```python
from build123d import *

# Parameters (mm, degrees)
BASE_W                = 83
BASE_H                = 80
MAIN_DEPTH            = 5
GEAR_AXIS_HOLES_D     = 5.8
CHAMFER1_SIZE         = 15
FILLET6_R             = 3
F_4_CLEARANCE_HOLE1_D = 3.2639


with BuildPart() as part:
    # Base → Main (new body)
    with BuildSketch(Plane.XY):
        with Locations((1.724154817, 0)):
            Rectangle(BASE_W, BASE_H)
    extrude(amount=MAIN_DEPTH)

    # Gear Axis Holes (through all)
    with Locations(Plane(origin=(0, 0, 5), x_dir=(-1, 0, 0), z_dir=(0, 0, 1))):
        with Locations((22.275845183, 20), (22.275845183, -20)):
            Hole(GEAR_AXIS_HOLES_D / 2)

    # Chamfer1
    chamfer1_edges = [part.edges().sort_by_distance(p)[0] for p in [
        (-39.775845183, -40, 2.5),
        (-39.775845183, 40, 2.5),
    ]]
    chamfer(chamfer1_edges, length=CHAMFER1_SIZE)

    # Fillet6
    fillet6_edges = [part.edges().sort_by_distance(p)[0] for p in [
        (-24.775845183, -40, 2.5),
        (-39.775845183, 25, 2.5),
        (-39.775845183, -25, 2.5),
        (-24.775845183, 40, 2.5),
        (43.224154817, 40, 2.5),
        (43.224154817, -40, 2.5),
    ]]
    fillet(fillet6_edges, radius=FILLET6_R)

    # #4 Clearance Hole1 (through all)
    with Locations(Plane.XY.offset(5)):
        with Locations((13.224154817, 35), (38.224154817, 35), (38.224154817, -35)):
            Hole(F_4_CLEARANCE_HOLE1_D / 2)


solid = part.part
```
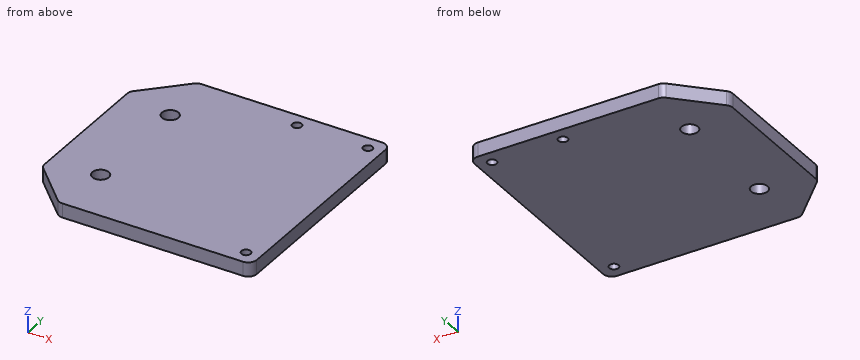
Design review of the part built by this model. Coordinates are the model's own, in mm. Round coordinates to 2 decimals unless told otherwise and drop trailing zeros. Write each loop counter-clockwise with the first axis right and the second up, starting at its lowest first coordinate (ties: lowest second). Pieces come first, ordered by that corner, then holes. Notation, with made-up numbers: (58.25, 69.5) -> (101.25, 69.5) arc R23 cw to (101.25, 84.5) -> close; hole circle Ø6 at (58, -30). An arc over 180 degrees is marked (long way). Write item = value, one per line. Start each with the question number.
1) Take a section at A-A, the plane z = 0.9. State the section outline as (x, y) points.
2) Take a section at B-B, the plane y = 20. State the section outline as (x, z) points.
3) Clearance check with a flat-ended pin moving along its axis: pin 1 (3.5 mm diameter, centred on x = -22.28, y = 20, fed in from +Z). State where the tip first meets the part, or that it passes through.
4) Take a section at D-D, the plane y = -21. State the section outline as (x, z) points, plus the area to 3 significant figures.
5) Wall thickness on probe 1 along X at (y, z) = (20, 1.6); probe 2 along X at (y, z) = (-32, 2.95); probe 3 along X at (y, z) = (31.5, 1.65): over which ranges is each line inside the solid? List them lowest first. Write a range as from..to.
6) Take a section at C-C, the plane y = 35. State the section outline as (x, z) points, plus the area to 3 significant figures.
Results list:
q1.outline = (-39.78, -23.76) arc R3 ccw to (-38.9, -25.88) -> (-25.65, -39.12) arc R3 ccw to (-23.53, -40) -> (40.22, -40) arc R3 ccw to (43.22, -37) -> (43.22, 37) arc R3 ccw to (40.22, 40) -> (-23.53, 40) arc R3 ccw to (-25.65, 39.12) -> (-38.9, 25.88) arc R3 ccw to (-39.78, 23.76) -> close; hole circle Ø5.8 at (-22.28, -20); hole circle Ø5.8 at (-22.28, 20); hole circle Ø3.26 at (13.22, 35); hole circle Ø3.26 at (38.22, -35); hole circle Ø3.26 at (38.22, 35)
q2.outline = (-39.78, 0) -> (-25.18, 0) -> (-25.18, 5) -> (-39.78, 5) -> close; (-19.38, 0) -> (43.22, 0) -> (43.22, 5) -> (-19.38, 5) -> close
q3.pin_1 = through
q4.outline = (-39.78, 0) -> (-25, 0) -> (-25, 5) -> (-39.78, 5) -> close; (-19.55, 0) -> (43.22, 0) -> (43.22, 5) -> (-19.55, 5) -> close
q4.area = 388 mm²
q5.probe_1 = -39.78..-25.18, -19.38..43.22
q5.probe_2 = -32.78..43.22
q5.probe_3 = -33.28..43.22
q6.outline = (-29.78, 0) -> (11.59, 0) -> (11.59, 5) -> (-29.78, 5) -> close; (14.86, 0) -> (36.59, 0) -> (36.59, 5) -> (14.86, 5) -> close; (39.86, 0) -> (43.22, 0) -> (43.22, 5) -> (39.86, 5) -> close
q6.area = 332 mm²
